```python
from build123d import *

# Parameters (mm, degrees)
SKETCH_1_W          = 24
SKETCH_1_H          = 72
EXTRUDE_2_DEPTH     = 3
SKETCH_2_R          = 2.1
CUT_EXTRUDE_1_DEPTH = 3
CUT_EXTRUDE_2_DEPTH = 3
FILLET_1_R          = 2


with BuildPart() as part:
    # 草图1 → 凸台-拉伸2 (new body)
    with BuildSketch(Plane(origin=(0, 0, 0), x_dir=(1, 0, 0), z_dir=(0, 1, 0))):
        Rectangle(SKETCH_1_W, SKETCH_1_H)
    extrude(amount=EXTRUDE_2_DEPTH)

    # 草图2 → 切除-拉伸1 (cut)
    with BuildSketch(Plane(origin=(0, 3, 0), x_dir=(1, 0, 0), z_dir=(0, 1, 0))):
        with Locations(Location((-8, -32, 0), (0, 0, 270))):
            Circle(SKETCH_2_R)
        with Locations(Location((-8, -24, 0), (0, 0, 270))):
            Circle(SKETCH_2_R)
        with Locations(Location((-8, -16, 0), (0, 0, 270))):
            Circle(SKETCH_2_R)
        with Locations(Location((-8, -8, 0), (0, 0, 270))):
            Circle(SKETCH_2_R)
        with Locations(Location((-8, 0, 0), (0, 0, 270))):
            Circle(SKETCH_2_R)
        with Locations(Location((-8, 8, 0), (0, 0, 270))):
            Circle(SKETCH_2_R)
        with Locations(Location((-8, 16, 0), (0, 0, 270))):
            Circle(SKETCH_2_R)
        with Locations(Location((-8, 24, 0), (0, 0, 270))):
            Circle(SKETCH_2_R)
        with Locations(Location((-8, 32, 0), (0, 0, 270))):
            Circle(SKETCH_2_R)
        with Locations(Location((8, -24, 0), (0, 0, 90))):
            Circle(SKETCH_2_R)
        with Locations(Location((8, -16, 0), (0, 0, 90))):
            Circle(SKETCH_2_R)
        with Locations(Location((8, -8, 0), (0, 0, 90))):
            Circle(SKETCH_2_R)
        with Locations(Location((8, 0, 0), (0, 0, 90))):
            Circle(SKETCH_2_R)
        with Locations(Location((8, 8, 0), (0, 0, 90))):
            Circle(SKETCH_2_R)
        with Locations(Location((8, 16, 0), (0, 0, 90))):
            Circle(SKETCH_2_R)
        with Locations(Location((8, 24, 0), (0, 0, 90))):
            Circle(SKETCH_2_R)
        with Locations(Location((8, 32, 0), (0, 0, 90))):
            Circle(SKETCH_2_R)
        with Locations(Location((8, -32, 0), (0, 0, 90))):
            Circle(SKETCH_2_R)
        with Locations(Location((0, -32, 0), (0, 0, 90))):
            Circle(SKETCH_2_R)
        with Locations(Location((0, 32, 0), (0, 0, 270))):
            Circle(SKETCH_2_R)
    extrude(amount=-CUT_EXTRUDE_1_DEPTH, mode=Mode.SUBTRACT)

    # 草图3 → 切除-拉伸2 (cut)
    with BuildSketch(Plane(origin=(0, 3, 0), x_dir=(1, 0, 0), z_dir=(0, 1, 0))):
        with BuildLine():
            Line((-2.1, -24), (-2.1, 24))
            ThreePointArc((-2.1, 24), (0, 26.1), (2.1, 24))
            Line((2.1, 24), (2.1, -24))
            ThreePointArc((2.1, -24), (0, -26.1), (-2.1, -24))
        make_face()
    extrude(amount=-CUT_EXTRUDE_2_DEPTH, mode=Mode.SUBTRACT)

    # 圆角1
    fillet_1_edges = [part.edges().sort_by_distance(p)[0] for p in [
        (12, 1.5, 36),
        (-12, 1.5, 36),
        (-12, 1.5, -36),
        (12, 1.5, -36),
    ]]
    fillet(fillet_1_edges, radius=FILLET_1_R)


solid = part.part
```
The model under review builds one solid part; all positions refer to its coordinate system, in mm. A direction names the side the tool comes from. Round coordinates to 2 decimals unless told otherwise and drop trailing zeros. Loops run counter-clockwise (first coordinate to the right, second up) from the corner with the lowest first, then second, coordinate; pieces in that order, holes last. Notation, with made-up numbers: (41, -1.5) -> (56, -1.5) arc R23 cw to (56, 30.5) -> close; hole circle Ø7 at (6, -37). An arc over 180 degrees is marked (long way). Answer in a Markdown table with one row per item.
1) Consider section C-C, the plane y = 1.2. Count the separate pieces of the cut face and the enclosed holes in it, plus the area to 3 significant figures.
Taken from the geometry:
| item | result |
|---|---|
| separate pieces | 1 |
| enclosed holes | 21 |
| area | 1,230 mm² |
2) Consider section B-B, the plane x = 0. Write out the cut boundary in (y, z).
Taken from the geometry:
| item | result |
|---|---|
| outline | (0, -36) -> (3, -36) -> (3, -34.1) -> (0, -34.1) -> close; (0, -29.9) -> (3, -29.9) -> (3, -26.1) -> (0, -26.1) -> close; (0, 26.1) -> (3, 26.1) -> (3, 29.9) -> (0, 29.9) -> close; (0, 34.1) -> (3, 34.1) -> (3, 36) -> (0, 36) -> close |
3) Tool access review of faces 4 (the flat face through (-12, 1, 0)), 5 (the flat face through (-2.1, 2, 0)): name each direction out of +Z, -Z, +X, -X, +Y, -Y from which nothing blocks a thin tool from reaching the whole face with its end or side.
Taken from the geometry:
| item | result |
|---|---|
| face 4 | +Z, -Z, -X, +Y, -Y |
| face 5 | +Y, -Y |
4) Draft analysis for pull direction Z (two halves, no side actions). For faces 1 (the cylindrical face through (0, 1.5, 26.1)), 2 (the cylindrical face through (11.4, 1.52, -35.43)), 3 (the flat face through (12, 1, 0)), state which applies: pulls with the +Z half, pulls with the -Z half, needs draft (parallel to the pull), parting line crosses it, or undercut.
Taken from the geometry:
| item | result |
|---|---|
| face 1 | undercut |
| face 2 | pulls with the -Z half |
| face 3 | needs draft |
5) Consider section A-A, the plane z = 8. Write out the cut boundary in (x, y).
Taken from the geometry:
| item | result |
|---|---|
| outline | (-12, 0) -> (-10.1, 0) -> (-10.1, 3) -> (-12, 3) -> close; (-5.9, 0) -> (-2.1, 0) -> (-2.1, 3) -> (-5.9, 3) -> close; (2.1, 0) -> (5.9, 0) -> (5.9, 3) -> (2.1, 3) -> close; (10.1, 0) -> (12, 0) -> (12, 3) -> (10.1, 3) -> close |
6) Wall thickness on line 1 along X through (y, z) = (1.2, 8); line 2 along X through (y, z) = (1.5, 30.5); line 3 along X through (y, z) = (0.9, 19.5): over which ranges is each line inside the solid? List them lowest first.
Taken from the geometry:
| item | result |
|---|---|
| line 1 | x = -12 to -10.1, -5.9 to -2.1, 2.1 to 5.9, 10.1 to 12 |
| line 2 | x = -12 to -9.47, -6.53 to -1.47, 1.47 to 6.53, 9.47 to 12 |
| line 3 | x = -12 to -2.1, 2.1 to 12 |
